Geometry check sheet. Reference: the model listing, model coordinates, mm. Round coordinates to 2 decimals unless told otherwise and drop trailing zeros. Loops run counter-clockwise (first coordinate to the right, second up) from the corner with the lowest first, then second, coordinate; pieces in that order, holes last. Notation, with made-up numbers: M 77,44.25 L 103,44.25 A21 cw 103,74.25 Z; hole C 63,45.25 d3. An arc over 180 degrees is marked long. Answer in a Markdown table with one row per item. Add a question column.
Autodesk Inventor part; units mm, degrees
ref_plane "YZ Plane" through (0, 0, 0) normal (1, 0, 0) x (0, 1, 0)
ref_plane "XZ Plane" through (0, 0, 0) normal (0, 1, 0) x (-1, 0, 0)
ref_plane "XY Plane" through (0, 0, 0) normal (0, 0, 1) x (1, 0, 0)
sketch "Sketch1" plane through (0, 0, 0) normal (0, 1, 0) x (-1, 0, 0)
  line L0 (0, 0) -> (-584.2, 0)
  line L1 (-584.2, 0) -> (-584.2, -812.8)
  line L2 (-584.2, -812.8) -> (0, -812.8)
  line L3 (0, -812.8) -> (0, 0)
  dimension "d0" = 584.2
  dimension "d1" = 812.8
extrude "Extrusion1" add sketch "Sketch1" along normal blind 3.175
sketch "Sketch2" plane through (0, 0, 0) normal (0, -1, 0) x (1, 0, 0)
  line L0 (0, 0) -> (584.2, 0)
  line L1 (0, -812.8) -> (0, 0)
  line L2 (584.2, -812.8) -> (0, -812.8)
  line L3 (584.2, 0) -> (584.2, -812.8)
  line L4 (584.2, 0) -> (584.2, -812.8)
  line L5 (584.2, -323.85) -> (558.8, -323.85)
  line L6 (558.8, -323.85) -> (558.8, -488.95)
  line L7 (558.8, -488.95) -> (584.2, -488.95)
  line L8 (584.2, -488.95) -> (584.2, -323.85)
  line L9 (0, -812.8) -> (0, 0)
  line L10 (0, -323.85) -> (25.4, -323.85)
  line L11 (25.4, -323.85) -> (25.4, -488.95)
  line L12 (25.4, -488.95) -> (0, -488.95)
  line L13 (0, -488.95) -> (0, -323.85)
  line L14 (584.2, 0) -> (508, 0)
  line L15 (508, 0) -> (508, -234.95)
  line L16 (508, -234.95) -> (584.2, -234.95)
  line L17 (584.2, -234.95) -> (584.2, 0)
  line L18 (0, 0) -> (76.2, 0)
  line L19 (76.2, 0) -> (76.2, -234.95)
  line L20 (76.2, -234.95) -> (0, -234.95)
  line L21 (0, -234.95) -> (0, 0)
  line L22 (0, -812.8) -> (76.2, -812.8)
  line L23 (76.2, -812.8) -> (76.2, -577.85)
  line L24 (76.2, -577.85) -> (0, -577.85)
  line L25 (0, -577.85) -> (0, -812.8)
  line L26 (584.2, -812.8) -> (508, -812.8)
  line L27 (508, -812.8) -> (508, -577.85)
  line L28 (508, -577.85) -> (584.2, -577.85)
  line L29 (584.2, -577.85) -> (584.2, -812.8)
  line L30 (508, -234.95) -> (406.4, -234.95)
  line L31 (406.4, -234.95) -> (406.4, -139.7)
  line L32 (406.4, -139.7) -> (508, -139.7)
  line L33 (508, -139.7) -> (508, -234.95)
  line L34 (508, -577.85) -> (406.4, -577.85)
  line L35 (406.4, -577.85) -> (406.4, -673.1)
  line L36 (406.4, -673.1) -> (508, -673.1)
  line L37 (508, -673.1) -> (508, -577.85)
  line L38 (76.2, -577.85) -> (177.8, -577.85)
  line L39 (177.8, -577.85) -> (177.8, -673.1)
  line L40 (177.8, -673.1) -> (76.2, -673.1)
  line L41 (76.2, -673.1) -> (76.2, -577.85)
  line L42 (76.2, -234.95) -> (177.8, -234.95)
  line L43 (177.8, -234.95) -> (177.8, -139.7)
  line L44 (177.8, -139.7) -> (76.2, -139.7)
  line L45 (76.2, -139.7) -> (76.2, -234.95)
  dimension "d4" = 165.1
  dimension "d5" = 165.1
  dimension "d6" = 25.4
  dimension "d7" = 25.4
  dimension "d8" = 323.85
  dimension "d9" = 323.85
  dimension "d10" = 76.2
  dimension "d11" = 234.95
  dimension "d12" = 76.2
  dimension "d13" = 234.95
  dimension "d14" = 76.2
  dimension "d15" = 234.95
  dimension "d16" = 76.2
  dimension "d17" = 234.95
  dimension "d18" = 101.6
  dimension "d19" = 95.25
  dimension "d20" = 101.6
  dimension "d21" = 95.25
  dimension "d22" = 101.6
  dimension "d23" = 95.25
  dimension "d24" = 101.6
  dimension "d25" = 95.25
extrude "Extrusion2" cut sketch "Sketch2" against normal blind 3.175 contours L0 L19 L20 L1 | L0 L3 L16 L15 | L44 L43 L42 L19 | L10 L11 L12 L1 | L15 L30 L31 L32 | L24 L23 L2 L1 | L3 L7 L6 L5 | L38 L39 L40 L23 | L3 L2 L27 L28 | L27 L36 L35 L34
properties part number "polycarb base"
1) Cross-section at C-C, the plane z = -614.5. Record the boundary of the cut face in (x, y) (3 decimals).
2) Cross-section at D-D, the plane z = -761. Record the boundary of the cut face in (x, y) (3 decimals), plus the area to 3 significant figures.
3) Thickness scan on L1, parallel to Z at x = 431, y = 2.45; L2, parallel to X at y = 0.95, z = -487.5; L3, parallel to X at y = 2.95, z = -39. Record the ranges inside material, lowest first. Write a range as [from, to].
4) Cross-section at A-A, the plane x = 440. Record the boundary of the cut face in (y, z) (3 decimals), plus the area to 3 significant figures.
5) Go/stop test with flat-tipped pins: pin 1 (1 mm diameter, centred on y = 1.5, z = -198, fed in from -X); pin 2 (1.6 mm diameter, centred on y = 1, z = -394, fed in from -X); pin 3 (1 mm diameter, centred on y = 2, z = -724.5, fed in from +X). Record where each tip stops, or that it passes through.
6) Cross-section at B-B, the plane y = 0.5. Record the boundary of the cut face in (x, z).
Worked answers:
| question | item | result |
|---|---|---|
| 1 | outline | M 177.8,0 L 406.4,0 L 406.4,3.175 L 177.8,3.175 Z |
| 2 | outline | M 76.2,0 L 508,0 L 508,3.175 L 76.2,3.175 Z |
| 2 | area | 1,370 mm2 |
| 3 | L1 | z = [-812.8, -673.1], [-577.85, -234.95], [-139.7, 0] |
| 3 | L2 | x = [25.4, 558.8] |
| 3 | L3 | x = [76.2, 508] |
| 4 | outline | M 0,-812.8 L 3.175,-812.8 L 3.175,-673.1 L 0,-673.1 Z; M 0,-577.85 L 3.175,-577.85 L 3.175,-234.95 L 0,-234.95 Z; M 0,-139.7 L 3.175,-139.7 L 3.175,0 L 0,0 Z |
| 4 | area | 1,980 mm2 |
| 5 | pin 1 | stops at x = 177.8 |
| 5 | pin 2 | stops at x = 25.4 |
| 5 | pin 3 | stops at x = 508 |
| 6 | outline | M 0,-577.85 L 177.8,-577.85 L 177.8,-673.1 L 76.2,-673.1 L 76.2,-812.8 L 508,-812.8 L 508,-673.1 L 406.4,-673.1 L 406.4,-577.85 L 584.2,-577.85 L 584.2,-488.95 L 558.8,-488.95 L 558.8,-323.85 L 584.2,-323.85 L 584.2,-234.95 L 406.4,-234.95 L 406.4,-139.7 L 508,-139.7 L 508,0 L 76.2,0 L 76.2,-139.7 L 177.8,-139.7 L 177.8,-234.95 L 0,-234.95 L 0,-323.85 L 25.4,-323.85 L 25.4,-488.95 L 0,-488.95 Z |
